```python
from build123d import *

# Parameters (mm, degrees)
SKETCH1_W           = 25
SKETCH1_H           = 50
SKETCH1_R           = 3.4
BOSS_EXTRUDE1_DEPTH = 3
SKETCH2_W           = 50
SKETCH2_H           = 3
BOSS_EXTRUDE2_DEPTH = 8
SKETCH3_W           = 8
SKETCH3_H           = 50
BOSS_EXTRUDE3_DEPTH = 42
SKETCH4_R           = 2.65
CUT_EXTRUDE1_DEPTH  = 6.6
SKETCH5_R           = 5.802370205
CUT_EXTRUDE2_DEPTH  = 9
FILLET2_R           = 1
SKETCH6_R           = 12.6
BOSS_EXTRUDE4_DEPTH = 2
FILLET4_R           = 1
SKETCH8_R           = 1.589780168
SKETCH8_R_2         = 1.777428262
CUT_EXTRUDE3_DEPTH  = 10
SKETCH9_W           = 49.021678163
SKETCH9_H           = 20.976854622
CUT_EXTRUDE4_DEPTH  = 68.79439129
SKETCH10_R          = 1.4
CUT_EXTRUDE5_DEPTH  = 56.950783118


with BuildPart() as part:
    # Sketch1 → Boss-Extrude1 (new body)
    with BuildSketch(Plane(origin=(0, 0, 0), x_dir=(1, 0, 0), z_dir=(0, 1, 0))):
        with Locations((2.276951673, 11.384758364)):
            Rectangle(SKETCH1_W, SKETCH1_H)
        with Locations(Location((1.276951673, 11.384758364, 0), (0, 0, 270))):
            Circle(SKETCH1_R, mode=Mode.SUBTRACT)
    extrude(amount=BOSS_EXTRUDE1_DEPTH)

    # Sketch2 → Boss-Extrude2 (add)
    with BuildSketch(Plane.ZY.offset(10.223048327)):
        with Locations((-11.384758364, 1.5)):
            Rectangle(SKETCH2_W, SKETCH2_H)
    extrude(amount=BOSS_EXTRUDE2_DEPTH)

    # Sketch3 → Boss-Extrude3 (add)
    with BuildSketch(Plane.XZ):
        with Locations((-14.223048327, -11.384758364)):
            Rectangle(SKETCH3_W, SKETCH3_H)
    extrude(amount=BOSS_EXTRUDE3_DEPTH)

    # Sketch4 → Cut-Extrude1 (cut)
    with BuildSketch(Plane(origin=(0, 3, 0), x_dir=(1, 0, 0), z_dir=(0, 1, 0))):
        with Locations(Location((-14.223048327, 32.384758364, 0), (0, 0, 270))):
            Circle(SKETCH4_R)
        with Locations(Location((-14.223048327, -9.615241636, 0), (0, 0, 270))):
            Circle(SKETCH4_R)
    cut_extrude1 = extrude(amount=-CUT_EXTRUDE1_DEPTH, mode=Mode.SUBTRACT)

    # Mirror1: Cut-Extrude1 across plane
    add(cut_extrude1.mirror(Plane.ZX.offset(-19.5)), mode=Mode.SUBTRACT)

    # Sketch5 → Cut-Extrude2 (cut)
    with BuildSketch(Plane.ZY.offset(18.223048327)):
        with Locations((-11.836279124, -21)):
            Circle(SKETCH5_R)
    extrude(amount=-CUT_EXTRUDE2_DEPTH, mode=Mode.SUBTRACT)

    # Fillet2
    fillet2_edges = [part.edges().sort_by_distance(p)[0] for p in [
        (-10.223048327, -21, -17.638649329),
    ]]
    fillet(fillet2_edges, radius=FILLET2_R)

    # Mirror2: Cut-Extrude1 across plane
    add(cut_extrude1.mirror(Plane.ZY.offset(1.723048327)), mode=Mode.SUBTRACT)

    # Sketch6 → Boss-Extrude4 (add)
    with BuildSketch(Plane(origin=(0, 3, 0), x_dir=(1, 0, 0), z_dir=(0, 1, 0))):
        with BuildLine():
            Line((14.776951673, 5.825082115), (14.776951673, 16.944434614))
            ThreePointArc((14.776951673, 16.944434614), (-13.323048327, 11.384758364), (14.776951673, 5.825082115))
        make_face()
        with Locations(Location((1.276951673, 11.384758364, 0), (0, 0, 270))):
            Circle(SKETCH6_R, mode=Mode.SUBTRACT)
    extrude(amount=BOSS_EXTRUDE4_DEPTH)

    # Fillet4
    # the kernel refuses this fillet: 1 mm, written as the material it takes off along each edge
    with BuildSketch(Plane(origin=(14.776951673, 5, -3.325082115), x_dir=(0, -1, 0), z_dir=(0, 0, -1))) as fillet4_piece_1:
        with BuildLine():
            CenterArc((FILLET4_R, FILLET4_R), FILLET4_R, 180, 90)
            Line((0, FILLET4_R), (0, 0))
            Line((0, 0), (FILLET4_R, 0))
        make_face()
    extrude(amount=16.119352499, mode=Mode.SUBTRACT)

    # Sketch8 → Cut-Extrude3 (cut)
    with BuildSketch(Plane(origin=(0, 3, 0), x_dir=(1, 0, 0), z_dir=(0, 1, 0))):
        with Locations(Location((1.276951673, 19.884758364, 0), (0, 0, 270))):
            Circle(SKETCH8_R)
        with Locations(Location((1.276951673, 2.884758364, 0), (0, 0, 270))):
            Circle(SKETCH8_R_2)
    extrude(amount=-CUT_EXTRUDE3_DEPTH, mode=Mode.SUBTRACT)

    # Sketch9 → Cut-Extrude4 (cut, through all)
    with BuildSketch(Plane.XY.offset(13.615241636)):
        with Locations((-9.733887409, 10.488427311)):
            Rectangle(SKETCH9_W, SKETCH9_H)
    extrude(amount=-CUT_EXTRUDE4_DEPTH, mode=Mode.SUBTRACT)

    # Sketch10 → Cut-Extrude5 (cut, through all)
    with BuildSketch(Plane(origin=(0, -3.6, 0), x_dir=(1, 0, 0), z_dir=(0, 1, 0))):
        with Locations(Location((-14.223048327, 32.384758364, 0), (0, 0, 270))):
            Circle(SKETCH10_R)
    cut_extrude5 = extrude(amount=-CUT_EXTRUDE5_DEPTH, mode=Mode.SUBTRACT)

    # Mirror3: Cut-Extrude5 across plane
    add(cut_extrude5.mirror(Plane.XY.offset(-11.384758364)), mode=Mode.SUBTRACT)


solid = part.part
```
Input: part model. Units: mm. Frame: model coordinates. A direction names the side the tool comes from. Coordinates: 2 decimals unless noted, no trailing zeros. Write each loop counter-clockwise with the first axis right and the second up, starting at its lowest first coordinate (ties: lowest second). Pieces come first, ordered by that corner, then holes.
1) Pin query (flat end, axial travel): pin 1 Ø3 at (x, z) = (-14.22, -32.38) entering from -Y; pin 2 Ø2.5 at (x, z) = (-15, -31.5) entering from +Y. Return the tip coordinate at first contact, or that it passes through.
2) Set-up query: faces 4 (the flat face through (-18.223, -16, -17)), 5 (the flat face through (-15, -3.6, -31)), 6 (the flat face through (-15, -35.4, -31)). Return all of +Z, -Z, +X, -X, +Y, -Y with unobstructed straight access to the full face (end or side cutting, diameter ignored); none if empty.
3) Section B-B on x = -17.5. Output: boundary loops of the cut face in (y, z).
4) Section C-C on y = -33. Output: boundary loops of the cut face in (x, z), and give its area (3 significant figures).
5) Mould query, pull axis Z, two halves, no side actions, for faces 1 (the cylindrical face through (-11.99, -1.77, -30.96)), 2 (the flat face through (-10.223, -16, -17)), 3 (the flat face through (-14, -21, -36.385)). Classes: pulls with the +Z half, pulls with the -Z half, needs draft (parallel to the pull), parting line crosses it, or undercut.
6) Material intervals for line 1 along Z through (x, y) = (-14.5, -30); line 2 along Y through (x, z) = (-10.75, -13); line 3 along Z through (x, y) = (-16.5, -24.5), sorted ascending.
7) Section A-A on y = -21. Output: boundary loops of the cut face in (x, z), and give its area (3 significant figures).
Check result:
1. pin 1: stops at y = -35.4
1. pin 2: stops at y = -3.6
2. face 4: +Z, -Z, -X, +Y, -Y
2. face 5: +Y
2. face 6: -Y
3. outline: (-42, -36.38) - (0, -36.38) - (0, 13.62) - (-42, 13.62) - close; hole circle Ø11.6 at (-21, -11.84)
4. outline: (-18.22, -36.38) - (-10.22, -36.38) - (-10.22, 13.62) - (-18.22, 13.62) - close; hole circle Ø2.8 at (-14.22, -32.38); hole circle Ø2.8 at (-14.22, 9.62)
4. area: 388 mm2
5. face 1: undercut
5. face 2: needs draft
5. face 3: pulls with the -Z half
6. line 1: z = -36.38 to -33.76, -31.01 to 8.24, 10.99 to 13.62
6. line 2: y = -42 to -26.81, -15.19 to 0
6. line 3: z = -36.38 to -16.46, -7.21 to 13.62
7. outline: (-18.22, -36.38) - (-10.22, -36.38) - (-10.22, -18.64) arc R1 ccw to (-11.22, -17.64) - (-18.22, -17.64) - close; (-18.22, -6.03) - (-11.22, -6.03) arc R1 ccw to (-10.22, -5.03) - (-10.22, 13.62) - (-18.22, 13.62) - close; hole circle Ø2.8 at (-14.22, -32.38); hole circle Ø2.8 at (-14.22, 9.62)
7. area: 294 mm2
